Input: part model. Units: mm. Frame: model coordinates. Face numbers are marked on the shaded views. A direction names the side the tool comes from. Coordinates: 2 decimals unless noted, no trailing zeros. Write each loop counter-clockwise with the first axis right and the second up, starting at its lowest first coordinate (ties: lowest second). Pieces come first, ordered by that corner, then holes. Notation, with made-up numbers: (70.5, 65.5) - (96.5, 65.5) arc R11 cw to (96.5, 77.5) - close; hole circle Ø10 at (10.25, -28). An arc over 180 degrees is marked (long way). Put each result on its own line as item: value. Start each with the question number.
1. Pin query (flat end, axial travel): pin 1 (3 mm diameter, centred on x = 25, z = -5, fed in from +Y); pin 2 (3 mm diameter, centred on x = 15.5, y = -6.5, fed in from +Z); pin 3 (3 mm diameter, centred on y = 1, z = 7, fed in from +X); pin 4 (4.5 mm diameter, centred on y = -1.5, z = -1.5, fed in from -X). Return the tip coordinate at first contact, or that it passes through.
2. Access query for the marked faces 3 and 4. Directions: +Z, -Z, +X, -X, +Y, -Y. A direction counts if a zero-diameter tool reaches every point of the face in a straight line with its end or side. Return the directions, or none.
3. Cut plane A-A, the plane x = 26.5. Return loops of the section in (y, z).
4. Pull-direction query (Z, two-part tool) for the marked faces 1 and 2; classes: released by +Z, released by -Z, zero draft, split by the parting line, or undercut.
5. Cut plane B-B, the plane z = 8.5. Return loops of the section in (x, y).
6. Line query: line 1 (Y direction, x = 32.5, z = -6); line 2 (X direction, y = -6.25, z = 9); line 3 (X direction, y = -12, z = -5). Output: solid intervals per line, ascending.
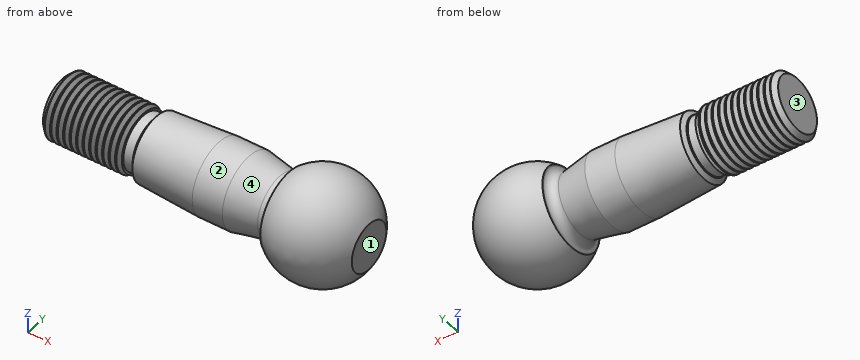
from build123d import *


with BuildPart() as part:
    # Çizim1 → Döndür2 (revolve)
    with BuildSketch(Plane.XY, mode=Mode.PRIVATE) as d_nd_r2_sk:
        with BuildLine():
            Line((58.889857915, -5.151471863), (58.889857915, -0.572124064))
            ThreePointArc((58.889857915, -0.572124064), (51.925602912, 4.66137958), (43.5, 2.447870214))
            Line((43.5, 2.447870214), (43.5, 2.171445263))
            ThreePointArc((43.5, 2.171445263), (42.95411733, 1.014008388), (41.713786507, 0.699004488))
            Line((41.713786507, 0.699004488), (35.8, 1.848528137))
            Line((35.8, 1.848528137), (30, 1.848528137))
            Line((30, 1.848528137), (18, 1.148528137))
            Line((18, 1.148528137), (17.451517244, 0.198528137))
            Line((17.451517244, 0.198528137), (17.278312164, 0.098528137))
            Line((17.278312164, 0.098528137), (15.5, 0.098528137))
            Line((15.5, 0.098528137), (15.5, 0.508911637))
            Line((15.5, 0.508911637), (15.205329949, -0.001471863))
            Line((15.205329949, -0.001471863), (14.71458222, 0.848528137))
            Line((14.71458222, 0.848528137), (14.446077678, 0.848528137))
            Line((14.446077678, 0.848528137), (13.955329949, -0.001471863))
            Line((13.955329949, -0.001471863), (13.46458222, 0.848528137))
            Line((13.46458222, 0.848528137), (13.196077678, 0.848528137))
            Line((13.196077678, 0.848528137), (12.705329949, -0.001471863))
            Line((12.705329949, -0.001471863), (12.21458222, 0.848528137))
            Line((12.21458222, 0.848528137), (11.946077678, 0.848528137))
            Line((11.946077678, 0.848528137), (11.455329949, -0.001471863))
            Line((11.455329949, -0.001471863), (10.96458222, 0.848528137))
            Line((10.96458222, 0.848528137), (10.696077678, 0.848528137))
            Line((10.696077678, 0.848528137), (10.205329949, -0.001471863))
            Line((10.205329949, -0.001471863), (9.71458222, 0.848528137))
            Line((9.71458222, 0.848528137), (9.446077678, 0.848528137))
            Line((9.446077678, 0.848528137), (8.955329949, -0.001471863))
            Line((8.955329949, -0.001471863), (8.46458222, 0.848528137))
            Line((8.46458222, 0.848528137), (8.196077678, 0.848528137))
            Line((8.196077678, 0.848528137), (7.705329949, -0.001471863))
            Line((7.705329949, -0.001471863), (7.21458222, 0.848528137))
            Line((7.21458222, 0.848528137), (6.946077678, 0.848528137))
            Line((6.946077678, 0.848528137), (6.455329949, -0.001471863))
            Line((6.455329949, -0.001471863), (5.96458222, 0.848528137))
            Line((5.96458222, 0.848528137), (5.696077678, 0.848528137))
            Line((5.696077678, 0.848528137), (5.205329949, -0.001471863))
            Line((5.205329949, -0.001471863), (4.71458222, 0.848528137))
            Line((4.71458222, 0.848528137), (4.446077678, 0.848528137))
            Line((4.446077678, 0.848528137), (3.955329949, -0.001471863))
            Line((3.955329949, -0.001471863), (3.46458222, 0.848528137))
            Line((3.46458222, 0.848528137), (3.196077678, 0.848528137))
            Line((3.196077678, 0.848528137), (2.705329949, -0.001471863))
            Line((2.705329949, -0.001471863), (2.21458222, 0.848528137))
            Line((2.21458222, 0.848528137), (1.946077678, 0.848528137))
            Line((1.946077678, 0.848528137), (1.455329949, -0.001471863))
            Line((1.455329949, -0.001471863), (0.96458222, 0.848528137))
            Line((0.96458222, 0.848528137), (0.848528137, 0.848528137))
            Line((0.848528137, 0.848528137), (0, 0))
            Line((0, 0), (0, -5.151471863))
            Line((0, -5.151471863), (6, -5.151471863))
            Line((6, -5.151471863), (7.6, -5.151471863))
            Line((7.6, -5.151471863), (58.889857915, -5.151471863))
        make_face()
    revolve(d_nd_r2_sk.sketch.rotate(Axis((0, -5.151471863, 0), (1, 0, 0)), 180), axis=Axis((0, -5.151471863, 0), (1, 0, 0)))


solid = part.part
Report:
1. pin 1: stops at y = 0.58
1. pin 2: stops at z = 6
1. pin 3: stops at x = 56.23
1. pin 4: stops at x = 0
2. face 3: +Z, -Z, -X, +Y, -Y
2. face 4: none
3. outline: circle Ø13.59 at (-5.15, 0)
4. face 1: zero draft
4. face 2: split by the parting line
5. outline: circle Ø10.54 at (50, -5.15)
6. line 1: y = -8.76 to -1.55
6. line 2: x = 45.78 to 54.22
6. line 3: x = 44.7 to 55.3
